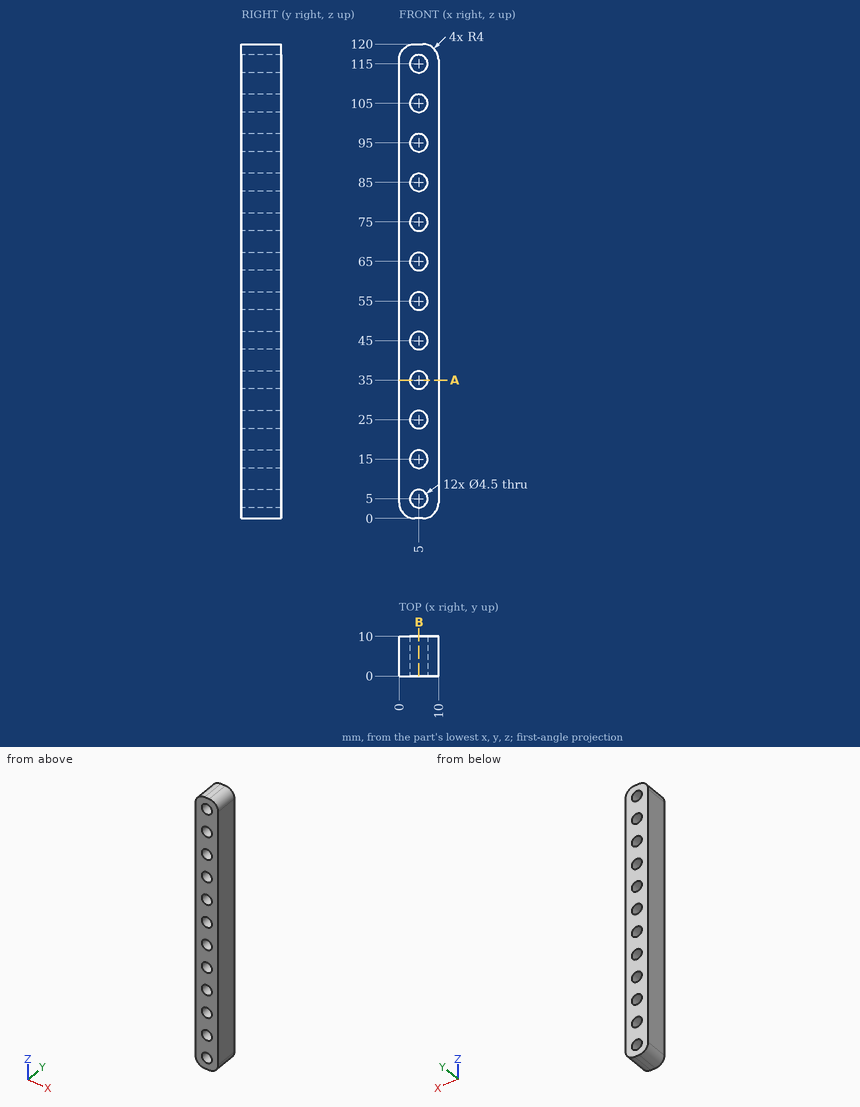
Design review of the part shown in the three views and the two pictorial views. Dimensions are in mm from the part's minimum x, y and z. Give positions to 0.01 mm unless a question says otherwise; leave off trailing zeros. Loops run counter-clockwise (first coordinate to the right, second up) from the corner with the lowest first, then second, coordinate; pieces in that order, holes last. Notation, with made-up numbers: (24, 53) - (78, 53) arc R24 cw to (78, 70) - close; hole circle Ø3 at (57, 25). An arc over 180 degrees is marked (long way). Write item = value, one per line.
1) Take a section at A-A on z = 35. State the section outline as (x, y) points, and give its area (3 significant figures).
Result sheet:
outline = (0, 0) - (2.75, 0) - (2.75, 10) - (0, 10) - close; (7.25, 0) - (10, 0) - (10, 10) - (7.25, 10) - close
area = 55.0 mm2
2) To check wall thickness, follow line 1 (X direction, y = 5, z = 115); line 2 (X direction, y = 7.5, z = 54); line 3 (Z direction, x = 9.25, y = 7). State the ranges of each line that lie inside material, in increasing order.
Result sheet:
line_1 = 0 to 2.75, 7.25 to 10
line_2 = 0 to 2.98, 7.02 to 10
line_3 = 1.67 to 118.33
3) Clearance check with flat-ended pins moving along their axes: pin 1 Ø4 at (x, z) = (5, 95) entering from +Y; pin 2 Ø4 at (x, y) = (1, 6.5) entering from -Z. State where each tip first meets the part, or that it passes through.
Result sheet:
pin_1 = through
pin_2 = 0.13
4) Take a section at B-B on x = 5. Count the separate pieces of the cut face and the enclosed holes in it, and give its area (3 significant figures).
Result sheet:
separate_pieces = 13
enclosed_holes = 0
area = 660 mm2
